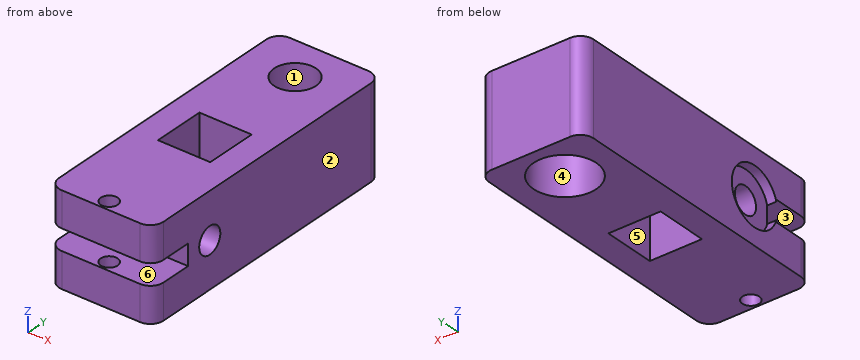
from build123d import *

# Parameters (mm, degrees)
CROQUIS1_R              = 12
CROQUIS1_R_2            = 3.25
SALIENTE_EXTRUIR1_DEPTH = 35
SALIENTE_EXTRUIR2_START = -10
CROQUIS2_R              = 12
CROQUIS2_R_2            = 8
SALIENTE_EXTRUIR2_DEPTH = 10
CROQUIS3_R              = 5.1
CROQUIS3_W              = 8
CROQUIS3_H              = 16.86
CORTAR_EXTRUIR2_DEPTH   = 123.321007599
CROQUIS4_R              = 11
CORTAR_EXTRUIR3_DEPTH   = 3.5


with BuildPart() as part:
    # Croquis1 → Saliente-Extruir1 (new body)
    # profile 1 of 2: a face of its own
    with BuildSketch(Plane.XY):
        with BuildLine():
            Line((0, 105.17), (0, 40.17))
            Line((0, 40.17), (10, 40.17))
            Line((10, 40.17), (10, 60.17))
            Line((10, 60.17), (30, 60.17))
            Line((30, 60.17), (30, 40.17))
            Line((30, 40.17), (40, 40.17))
            Line((40, 40.17), (40, 105.17))
            ThreePointArc((40, 105.17), (38.535533906, 108.705533906), (35, 110.17))
            Line((35, 110.17), (5, 110.17))
            ThreePointArc((5, 110.17), (1.464466094, 108.705533906), (0, 105.17))
        make_face()
        with Locations((20, 93.74)):
            Circle(CROQUIS1_R, mode=Mode.SUBTRACT)
    # profile 2 of 2: a face of its own
    with BuildSketch(Plane.XY):
        with BuildLine():
            Line((5, 0), (35, 0))
            ThreePointArc((35, 0), (38.535533906, 1.464466094), (40, 5))
            Line((40, 5), (40, 40.17))
            Line((40, 40.17), (0, 40.17))
            Line((0, 40.17), (0, 5))
            ThreePointArc((0, 5), (1.464466094, 1.464466094), (5, 0))
        make_face()
        with Locations((20, 4)):
            Circle(CROQUIS1_R_2, mode=Mode.SUBTRACT)
    extrude(amount=SALIENTE_EXTRUIR1_DEPTH)

    # Croquis2 → Saliente-Extruir2 (add)
    with BuildSketch(Plane.XY.offset(35).offset(SALIENTE_EXTRUIR2_START)):
        with Locations((20, 93.74)):
            Circle(CROQUIS2_R)
        with Locations((20, 93.74)):
            Circle(CROQUIS2_R_2, mode=Mode.SUBTRACT)
    extrude(amount=SALIENTE_EXTRUIR2_DEPTH)

    # Croquis3 → Cortar-Extruir2 (cut, through all)
    with BuildSketch(Plane.ZY):
        with Locations((17.5, 27.36)):
            Circle(CROQUIS3_R)
        with Locations((17.5, 8.43)):
            Rectangle(CROQUIS3_W, CROQUIS3_H)
    extrude(amount=-CORTAR_EXTRUIR2_DEPTH, mode=Mode.SUBTRACT)

    # Croquis4 → Cortar-Extruir3 (cut)
    with BuildSketch(Plane.ZY):
        with Locations((17.5, 27.36)):
            Circle(CROQUIS4_R)
    extrude(amount=-CORTAR_EXTRUIR3_DEPTH, mode=Mode.SUBTRACT)


solid = part.part
Could you check a few things on this model? Use its own coordinates, in mm. Face numbers are marked on the shaded views. A direction names the side the tool comes from. Coordinates: 2 decimals unless noted, no trailing zeros. Write each loop counter-clockwise with the first axis right and the second up, starting at its lowest first coordinate (ties: lowest second). Pieces come first, ordered by that corner, then holes. Notation, with made-up numbers: (43.25, 25.5) - (61.25, 25.5) arc R21 cw to (61.25, 31.5) - close; hole circle Ø4 at (-38, -6). An arc over 180 degrees is marked (long way). Put each result on its own line as item: value. Start each with the question number.
Q1. Which directions (+Z, -Z, +X, -X, +Y, -Y) give clear straight access to the entire face, cutting with the end or side of a thin tool? Please do the marked faces 4, 5 and 6.
Q2. Thinking about a two-plate mould opening in X: for the marked faces 1, 2 and 3, which applies, pulls with the +X half, pulls with the -X half, needs draft (parallel to the pull), parting line crosses it, or undercut?
Q3. I want a section at D-D on z = 10. Write out the boundary of the cut face in (x, y).
Q4. I'm going to push flat-ended pins straight in: P1, Ø6.5, axis at y = 30.5, z = 12.5, coming from the -X side; P2, Ø2.5, axis at x = 22.5, z = 18, coming from the -Y side. Where does each tip first touch, or does it pass through?
Q5. I want a section at A-A on x = 20. Count the separate pieces of the cut face and the enclosed holes in it, plus the area to 3 significant figures.
Q6. I want a section at C-C on y = 93.74. Write out the boundary of the cut face in (x, z), plus the area to 3 significant figures.
Q7. Please list where these lines run through material, in increasing order: L1, parallel to Z at x = 10, y = 11; L2, parallel to Y at x = 20, z = 32; L3, parallel to Y at x = 14, z = 17.
Q8. I want a section at B-B on z = 17.5. Write out the boundary of the cut face in (x, y), plus the area to 3 significant figures.
Checks:
1. face 4: -Z
1. face 5: +Z, -Z
1. face 6: +X, -X, -Y
2. face 1: undercut
2. face 2: pulls with the +X half
2. face 3: needs draft
3. outline: (0, 5) arc R5 ccw to (5, 0) - (35, 0) arc R5 ccw to (40, 5) - (40, 105.17) arc R5 ccw to (35, 110.17) - (5, 110.17) arc R5 ccw to (0, 105.17) - (0, 35.41) - (3.5, 35.41) - (3.5, 19.31) - (0, 19.31) - close; hole circle Ø24 at (20, 93.74); hole (10, 40.17) - (30, 40.17) - (30, 60.17) - (10, 60.17) - close; hole circle Ø6.5 at (20, 4)
4. P1: x = 3.5
4. P2: y = 16.86
5. separate pieces: 5
5. enclosed holes: 1
5. area: 2,000 mm²
6. outline: (0, 0) - (8, 0) - (8, 25) - (12, 25) - (12, 35) - (0, 35) - close; (28, 25) - (32, 25) - (32, 0) - (40, 0) - (40, 35) - (28, 35) - close
6. area: 640 mm²
7. L1: 0 to 13.5, 21.5 to 35
7. L2: 0 to 0.75, 7.25 to 40.17, 60.17 to 85.74, 101.74 to 110.17
7. L3: 16.86 to 22.28, 32.44 to 40.17, 60.17 to 83.35, 104.13 to 110.17
8. outline: (0, 38.36) - (3.5, 38.36) - (3.5, 32.46) - (40, 32.46) - (40, 105.17) arc R5 ccw to (35, 110.17) - (5, 110.17) arc R5 ccw to (0, 105.17) - close; (3.5, 16.86) - (40, 16.86) - (40, 22.26) - (3.5, 22.26) - close; hole circle Ø24 at (20, 93.74); hole (10, 40.17) - (30, 40.17) - (30, 60.17) - (10, 60.17) - close
8. area: 2,420 mm²
